Here's how the part is built. I have some questions about the finished solid (model axes, mm). A direction names the side the tool comes from. Coordinates: 2 decimals unless noted, no trailing zeros. Write each loop counter-clockwise with the first axis right and the second up, starting at its lowest first coordinate (ties: lowest second). Pieces come first, ordered by that corner, then holes. Notation, with made-up numbers: (-15.75, -7) -> (-10.75, -7) arc R34 cw to (-10.75, 30) -> close; hole circle Ø2 at (71.5, 43). An arc over 180 degrees is marked (long way). Put each result on its own line as item: value.
```python
from build123d import *

# Parameters (mm, degrees)
F0_R     = 26
F1_DEPTH = 2
F2_R     = 22.5
F3_DEPTH = 2
F5_DEPTH = 2
F6_R     = 15
F7_DEPTH = 5


with BuildPart() as f1:
    # F0 (on Top) → F1 (new body)
    with BuildSketch(Plane.XY):
        Circle(F0_R)
    extrude(amount=F1_DEPTH)

    # F2 (on face) → F3 (join)
    with BuildSketch(Plane.XY.offset(2)):
        Circle(F2_R)
    extrude(amount=F3_DEPTH)

    # F4 (on face) → F5 (join)
    with BuildSketch(Plane.XY.offset(4)):
        with BuildLine():
            Line((-22.3533584706, -1.8999999156), (-22.3533584706, 2.5002909302))
            Line((-22.3533584706, 2.5002909302), (-22.3606472461, 2.5002909302))
            ThreePointArc((-22.3606472461, 2.5002909302), (-22.4979786383, 0.3015911014), (-22.4196342593, -1.8999999156))
            Line((-22.4196342593, -1.8999999156), (-22.3533584706, -1.8999999156))
        make_face()
        with BuildLine():
            Line((-22.3606472461, 2.5002909302), (-22.3533584706, 2.5002909302))
            Line((-22.3533584706, 2.5002909302), (-22.3533584706, -1.8999999156))
            Line((-22.3533584706, -1.8999999156), (-22.4196342593, -1.8999999156))
            ThreePointArc((-22.4196342593, -1.8999999156), (0, -22.5), (22.4196342593, -1.8999999156))
            Line((22.4196342593, -1.8999999156), (22.4196342593, 1.8999999156))
            ThreePointArc((22.4196342593, 1.8999999156), (0.3015911015, 22.4979786383), (-22.3606472461, 2.5002909302))
        make_face()
        with BuildLine():
            ThreePointArc((-22.4196342593, -1.8999999156), (-22.4979786383, 0.3015911014), (-22.3606472461, 2.5002909302))
            Line((-22.3606472461, 2.5002909302), (-24.011714384, 2.5002909302))
            Line((-24.011714384, 2.5002909302), (-24.011714384, -1.8999999156))
            Line((-24.011714384, -1.8999999156), (-22.4196342593, -1.8999999156))
        make_face()
        with BuildLine():
            ThreePointArc((22.5, 0), (22.4798995865, 0.9508494008), (22.4196342593, 1.8999999156))
            Line((22.4196342593, 1.8999999156), (22.4196342593, -1.8999999156))
            ThreePointArc((22.4196342593, -1.8999999156), (22.4798995865, -0.9508494008), (22.5, 0))
        make_face()
        with BuildLine():
            Line((22.4196342593, 2.5002909302), (22.4196342593, 1.8999999156))
            ThreePointArc((22.4196342593, 1.8999999156), (22.4798995865, 0.9508494008), (22.5, 0))
            ThreePointArc((22.5, 0), (22.4798995865, -0.9508494008), (22.4196342593, -1.8999999156))
            Line((22.4196342593, -1.8999999156), (23.8429448439, -1.8999999156))
            Line((23.8429448439, -1.8999999156), (23.8429448439, 2.5002909302))
            Line((23.8429448439, 2.5002909302), (22.4196342593, 2.5002909302))
        make_face()
    extrude(amount=F5_DEPTH)

    # F6 (on face) → F7 (join)
    with BuildSketch(Plane.XY.offset(6)):
        Circle(F6_R)
    extrude(amount=F7_DEPTH)


solid = f1.part
```
Item 1: Imagine slicing it at B-B on z = 5. Write out the boundary of the cut face in (x, y).
Output:
outline: (-24.01, -1.9) -> (-22.42, -1.9) arc R22.5 ccw to (22.42, -1.9) -> (23.84, -1.9) -> (23.84, 2.5) -> (22.42, 2.5) -> (22.42, 1.9) arc R22.5 ccw to (-22.36, 2.5) -> (-24.01, 2.5) -> close
Item 2: If we mould it in two halves opening along Z, with no side actions, what happens to faces 4 (the flat face through (0, 0, 0)), 5 (the flat face through (23, 0, 4)), 6 (the flat face through (23.843, 0, 5))? For each: released by +Z, released by -Z, zero draft, split by the parting line, or undercut.
Output:
face 4: released by -Z
face 5: undercut
face 6: zero draft
Item 3: Imagine slicing it at C-C on y = 0. Write out the boundary of the cut face in (x, z), then the cut area to 3 significant figures.
Output:
outline: (-26, 0) -> (26, 0) -> (26, 2) -> (22.5, 2) -> (22.5, 4) -> (23.84, 4) -> (23.84, 6) -> (15, 6) -> (15, 11) -> (-15, 11) -> (-15, 6) -> (-24.01, 6) -> (-24.01, 4) -> (-22.5, 4) -> (-22.5, 2) -> (-26, 2) -> close
area: 440 mm²
Item 4: Imagine slicing it at D-D on y = 17.5. Write out the boundary of the cut face in (x, z), then the cut area to 3 significant figures.
Output:
outline: (-19.23, 0) -> (19.23, 0) -> (19.23, 2) -> (14.14, 2) -> (14.14, 6) -> (-14.14, 6) -> (-14.14, 2) -> (-19.23, 2) -> close
area: 190 mm²
Item 5: Which directions (+Z, -Z, +X, -X, +Y, -Y) give clear straight access to the entire face, cutting with the end or side of a thin tool? Please do faces 1 (the flat face through (23, -1.9, 5)), 2 (the cylindrical face through (-14.985, 0.66, 8.465)), 3 (the flat face through (-23, -1.9, 5)).
Output:
face 1: +Z, +X, -Y
face 2: +Z
face 3: +Z, -X, -Y
Item 6: Imagine slicing it at A-A on x = 0. Write out the boundary of the cut face in (y, z).
Output:
outline: (-26, 0) -> (26, 0) -> (26, 2) -> (22.5, 2) -> (22.5, 6) -> (15, 6) -> (15, 11) -> (-15, 11) -> (-15, 6) -> (-22.5, 6) -> (-22.5, 2) -> (-26, 2) -> close
Item 7: For P1, Ø1.5, axis at y = 10, z = 9.5, coming from the -X side; P2, Ø0.6, axis at y = 1, z = 5, coming from the -X side; P3, Ø1.1, axis at x = 23, z = 5.5, coming from the -Y side, each with a flat end and sliding along its axis, tell me the tip position at first contact or that it passes through.
Output:
P1: stops at x = -11.81
P2: stops at x = -24.01
P3: stops at y = -1.9
Item 8: Please list where these lines run through material, in increasing order: line 1 along Z through (x, y) = (-19.5, -11); line 2 along Z through (x, y) = (-15.5, 19); line 3 along Y through (x, z) = (8, 9). Write a range as from..to.
Output:
line 1: z = 0..6
line 2: z = 0..2
line 3: y = -12.69..12.69
